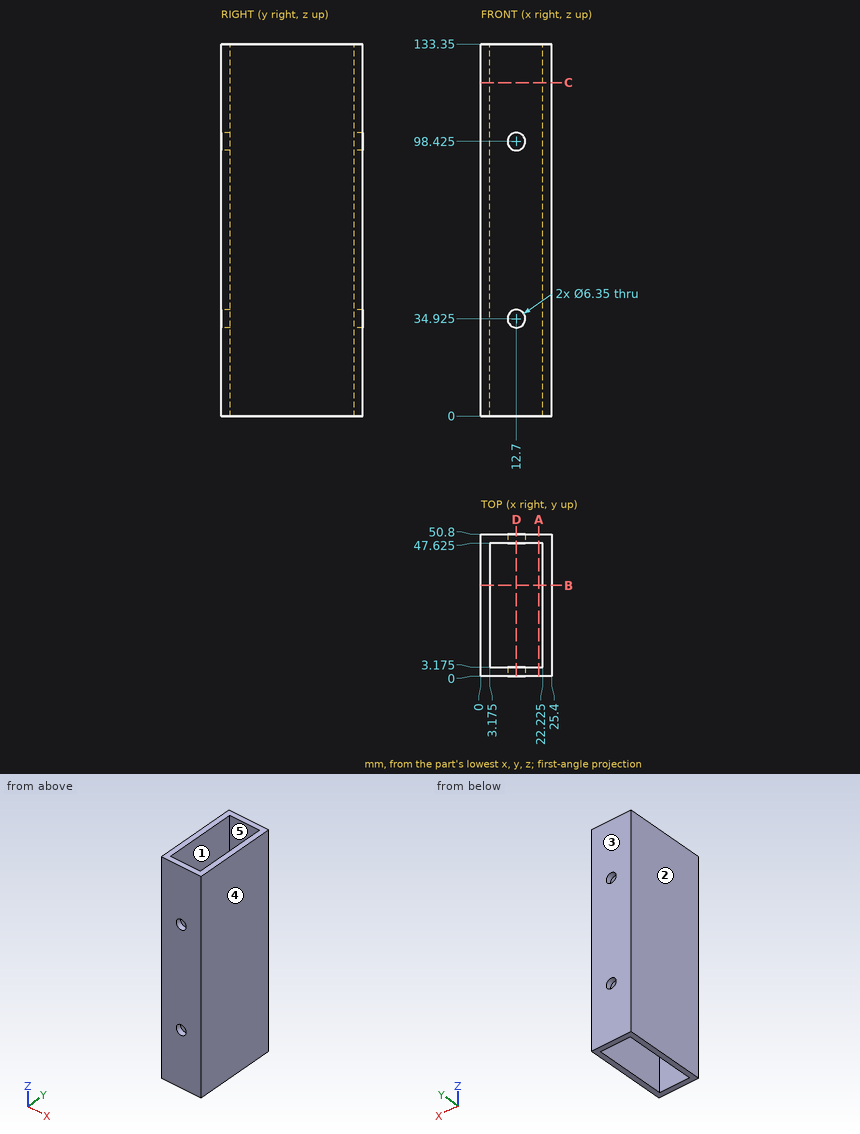
Input: dimensioned drawing with shaded views. Units: mm. Origin: part minimum x, y, z. A direction names the side the tool comes from. Coordinates: 2 decimals unless noted, no trailing zeros. Order: outer loops, then holes, each group sorted by start corner. A loop starts at its lowest first (then second) coordinate and runs counter-clockwise, first axis right, second up. Notation, with made-up numbers: (43, 40) - (56, 40) arc R26 ccw to (56, 74) - close; hole circle Ø4 at (-29.75, -16.75). An arc over 180 degrees is marked (long way). Return JSON: item names as keys, results as strings. Group by question number.
1. Pin query (flat end, axial travel): pin 1 (5 mm diameter, centred on x = 12.7, z = 98.425, fed in from -Y). Return the tip coordinate at first contact, or that it passes through.
2. Cut plane B-B (y = 32.5). Output: boundary loops of the cut face in (x, z) (3 decimals), plus the area to 3 significant figures.
3. Cut plane A-A (x = 20.75). Output: boundary loops of the cut face in (y, z) (3 decimals).
4. Pull-direction query (X, two-part tool) for the marked faces 1, 2 and 3; classes: pulls with the +X half, pulls with the -X half, needs draft (parallel to the pull), parting line crosses it, or undercut.
5. Cut plane D-D (x = 12.7). Output: boundary loops of the cut face in (y, z) (3 decimals).
6. Cut plane C-C (z = 119.5). Output: boundary loops of the cut face in (x, y) (3 decimals), plus the area to 3 significant figures.
7. Material intervals for line 1 along Y through (x, z) = (17, 14.5) (3 decimals); line 2 along X through (y, z) = (25, 20.5) (3 decimals), sorted ascending. Write a range as [from, to].
8. Set-up query: the marked faces 4 and 5. Return all of +Z, -Z, +X, -X, +Y, -Y with unobstructed straight access to the full face (end or side cutting, diameter ignored); none if empty.
Resolved:
{
 "1": {"pin 1": "passes through"},
 "2": {"outline": "(0, 0) - (3.175, 0) - (3.175, 133.35) - (0, 133.35) - close; (22.225, 0) - (25.4, 0) - (25.4, 133.35) - (22.225, 133.35) - close", "area": "847 mm²"},
 "3": {"outline": "(0, 0) - (3.175, 0) - (3.175, 133.35) - (0, 133.35) - close; (47.625, 0) - (50.8, 0) - (50.8, 133.35) - (47.625, 133.35) - close"},
 "4": {"face 1": "undercut", "face 2": "pulls with the -X half", "face 3": "needs draft"},
 "5": {"outline": "(0, 0) - (3.175, 0) - (3.175, 31.75) - (0, 31.75) - close; (0, 38.1) - (3.175, 38.1) - (3.175, 95.25) - (0, 95.25) - close; (0, 101.6) - (3.175, 101.6) - (3.175, 133.35) - (0, 133.35) - close; (47.625, 0) - (50.8, 0) - (50.8, 31.75) - (47.625, 31.75) - close; (47.625, 38.1) - (50.8, 38.1) - (50.8, 95.25) - (47.625, 95.25) - close; (47.625, 101.6) - (50.8, 101.6) - (50.8, 133.35) - (47.625, 133.35) - close"},
 "6": {"outline": "(0, 0) - (25.4, 0) - (25.4, 50.8) - (0, 50.8) - close; hole (3.175, 3.175) - (22.225, 3.175) - (22.225, 47.625) - (3.175, 47.625) - close", "area": "444 mm²"},
 "7": {"line 1": "y = [0, 3.175], [47.625, 50.8]", "line 2": "x = [0, 3.175], [22.225, 25.4]"},
 "8": {"face 4": "+Z, -Z, +X, +Y, -Y", "face 5": "+Z, -Z"}
}
